Work out the finished part from the listing and answer in its coordinate system (mm). A direction names the side the tool comes from. Give positions to 0.01 mm unless a question says otherwise; leave off trailing zeros. Loops run counter-clockwise (first coordinate to the right, second up) from the corner with the lowest first, then second, coordinate; pieces in that order, holes last. Notation, with made-up numbers: (-30.5, -24.75) - (-7.5, -24.75) arc R24 ccw to (-7.5, -13.75) - close; hole circle Ø3 at (88, 10.5). An arc over 180 degrees is marked (long way). One line per question, with ' | ' between items. Start each with the question number.
1. Which of the six approach directions +Z, -Z, +X, -X, +Y, -Y give full straight-line access (tool end or side, diameter ignored) to faces 1 (the face through (-4.941, -4.676, 3.313)), 2 (the face through (5.7, 0, 3.3)), 3 (the face through (-5.7, 0, 3.3)), 4 (the face through (-3.46, 5.86, 3.31)), 5 (the face through (-2.44, 6.38, 3.31))?
2. This flat-tipped pin is pushed along its axis until it touches: pin 1 (4 mm diameter, centred on x = -4.5, z = 4.5, fed in from -Y). Where does it stop, or does it pass through?
3. Find the intervals of material crossed by line 1 (Y direction, x = 0, z = 3.25); line 2 (Y direction, x = 0, z = 5); line 3 (X direction, y = 6.75, z = 1.75), in increasing order.
4. Section D-D (x = 3.5) is taken. Determine the outline of the cut face in (y, z).
5. Section C-C (z = 9.25) is taken. Determine the outline of the cut face in (x, y).
6. Section A-A (x = 0) is taken. Determine the outline of the cut face in (y, z).
7. For a pull along X with two mould halves and no side action, classify faces 6 (the face through (0.573, -4.363, 8.248)), 7 (the face through (5.66, -3.78, 3.31)), 8 (the face through (6.48, 2.07, 3.31)), 9 (the face through (-2, 2, 9.82)) as released by +X, released by -X, zero draft, split by the parting line, or undercut.
8. Section B-B (y = 0) is taken. Determine the outline of the cut face in (x, z), plus the area to 3 significant figures.
from build123d import *

# Parameters (mm, degrees)
SKETCH1_R              = 5.7
MOTOR_GEAR_SHAPE_DEPTH = 6.72
MOTOR_START            = -6.72
MOTOR_GEAR_TOOTH_DEPTH = 6.72
MOTOR_GEAR_TEETH_COUNT = 14
MOTOR_GEAR_TEETH_ANGLE = 334.28577
SKETCH3_R              = 4.4
SKETCH3_R_2            = 2.35
MOTOR_GEAR_BOSS_DEPTH  = 3.1
SKETCH4_R              = 2.35
MOTOR_SHAFT_HOLE_DEPTH = 15.861806289
MOTOR_SHAFT_FLAT_DEPTH = 4.9


with BuildPart() as part:
    # Sketch1 → motor gear shape (new body)
    with BuildSketch(Plane.XY):
        Circle(SKETCH1_R)
    extrude(amount=MOTOR_GEAR_SHAPE_DEPTH)

    # Sketch2 → motor gear tooth (add)
    with BuildSketch(Plane.XY.offset(6.72).offset(MOTOR_START)):
        with BuildLine():
            Line((0.375, 7.941150735), (0.77, 5.647751765))
            ThreePointArc((0.77, 5.647751765), (0, 5.7), (-0.77, 5.647751765))
            Line((-0.77, 5.647751765), (-0.375, 7.941150735))
            ThreePointArc((-0.375, 7.941150735), (0, 7.95), (0.375, 7.941150735))
        make_face()
    motor_gear_tooth = extrude(amount=MOTOR_GEAR_TOOTH_DEPTH)

    # motor gear teeth: motor gear tooth ×14 about axis
    motor_gear_teeth_axis = Axis((0, 0, 0), (0, 0, -1))
    for i in range(1, MOTOR_GEAR_TEETH_COUNT):
        add(motor_gear_tooth.rotate(motor_gear_teeth_axis, i * MOTOR_GEAR_TEETH_ANGLE / (MOTOR_GEAR_TEETH_COUNT - 1)))

    # Sketch3 → motor gear boss (add)
    with BuildSketch(Plane.XY.offset(6.72)):
        with Locations(Location((0, 0, 0), (0, 0, 180))):
            Circle(SKETCH3_R)
        with Locations(Location((0, 0, 0), (0, 0, 180))):
            Circle(SKETCH3_R_2, mode=Mode.SUBTRACT)
    extrude(amount=MOTOR_GEAR_BOSS_DEPTH)

    # Sketch4 → motor shaft hole (cut, through all)
    with BuildSketch(Plane.XY.offset(9.82)):
        with Locations(Location((0, 0, 0), (0, 0, 180))):
            Circle(SKETCH4_R)
    extrude(amount=-MOTOR_SHAFT_HOLE_DEPTH, mode=Mode.SUBTRACT)

    # Sketch5 → motor shaft flat (add)
    with BuildSketch(Plane(origin=(0, 0, 0), x_dir=(-1, 0, 0), z_dir=(0, 0, -1))):
        with BuildLine():
            Line((-3.108054054, -1.25), (3.108054054, -1.25))
            ThreePointArc((3.108054054, -1.25), (0, -3.35), (-3.108054054, -1.25))
        make_face()
    extrude(amount=-MOTOR_SHAFT_FLAT_DEPTH)


solid = part.part
Conclusion:
1) face 1: +Z, -Z, -Y | face 2: +Z, -Z, +X | face 3: +Z, -Z, -X | face 4: +Z, -Z | face 5: +Z, -Z, +Y
2) pin 1: y = -7.32
3) line 1: -7.95 to -1.25, 2.35 to 7.95 | line 2: -7.95 to -2.35, 2.35 to 7.95 | line 3: -3.71 to -2.7, -0.58 to 0.58, 2.7 to 3.71
4) outline: (-7.14, 0) - (-6, 0) - (-6, 6.72) - (-7.14, 6.72) - close; (-4.5, 0) - (4.5, 0) - (4.5, 6.72) - (2.67, 6.72) - (2.67, 9.82) - (-2.67, 9.82) - (-2.67, 6.72) - (-4.5, 6.72) - close; (6, 0) - (7.14, 0) - (7.14, 6.72) - (6, 6.72) - close
5) outline: circle Ø8.8 at (0, 0); hole circle Ø4.7 at (0, 0)
6) outline: (-7.95, 0) - (-1.25, 0) - (-1.25, 4.9) - (-2.35, 4.9) - (-2.35, 9.82) - (-4.4, 9.82) - (-4.4, 6.72) - (-7.95, 6.72) - close; (2.35, 0) - (7.95, 0) - (7.95, 6.72) - (4.4, 6.72) - (4.4, 9.82) - (2.35, 9.82) - close
7) face 6: split by the parting line | face 7: released by +X | face 8: undercut | face 9: zero draft
8) outline: (-5.7, 0) - (-2.35, 0) - (-2.35, 9.82) - (-4.4, 9.82) - (-4.4, 6.72) - (-5.7, 6.72) - close; (2.35, 0) - (5.7, 0) - (5.7, 6.72) - (4.4, 6.72) - (4.4, 9.82) - (2.35, 9.82) - close | area: 57.7 mm²
